Study the drawing (mm; zero at the part's minimum x, y, z) and answer. A direction names the side the tool comes from. Coordinates: 2 decimals unless noted, no trailing zeros. Order: outer loops, then holes, each group sorted by start corner. A loop starts at its lowest first (then second) coordinate and runs counter-clockwise, first axis right, second up. Notation, with made-up numbers: (25.5, 6) - (80.5, 6) arc R25 ccw to (80.5, 19) - close; hole circle Ø11 at (45, 46). An arc over 180 degrees is marked (long way). Write item = value, one per line.
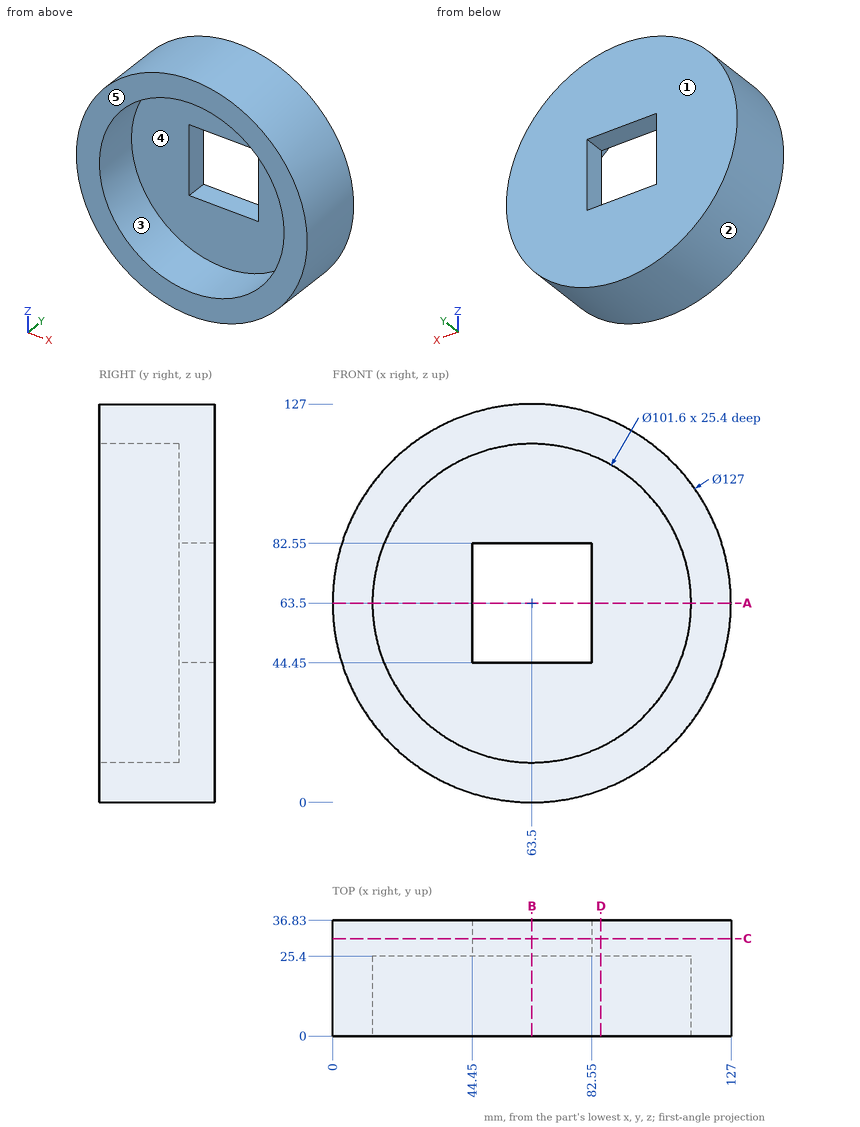
1) The part is cut by section A-A (z = 63.5). Determine the outline of the cut face in (x, y).
Returned:
outline = (0, 0) - (12.7, 0) - (12.7, 25.4) - (44.45, 25.4) - (44.45, 36.83) - (0, 36.83) - close; (82.55, 25.4) - (114.3, 25.4) - (114.3, 0) - (127, 0) - (127, 36.83) - (82.55, 36.83) - close
2) Straight lines are drawn through the part: line 1 along Z through (x, y) = (63.5, 11); line 2 along X through (y, z) = (12, 99). For each, find the intervals that lie inside material, in ascending order. Write a range as from..to.
Returned:
line_1 = 0..12.7, 114.3..127
line_2 = 10.85..27.16, 99.84..116.15
3) Flat-ended cylindrical pins translate along their axes: pin 1 Ø10 at (y, z) = (10, 51.5) entering from -X; pin 2 Ø3.5 at (y, z) = (28.5, 69.5) entering from -X; pin 3 Ø5.5 at (x, y) = (58.5, 33.5) entering from +Z. Find the tip coordinate at first contact, or state that the pin passes through.
Returned:
pin_1 = 0.39
pin_2 = 0.14
pin_3 = 126.96
4) For the marked faces 4 and 5, determine the directions among +Z, -Z, +X, -X, +Y, -Y from which every point of the face is accessible in a straight line to the end or side of a thin tool.
Returned:
face_4 = -Y
face_5 = +Z, -Z, +X, -X, -Y
5) Determine the mould class of the marked faces 1, 2 and 3 for opening direction X: pulls with the +X half, pulls with the -X half, needs draft (parallel to the pull), parting line crosses it, or undercut.
Returned:
face_1 = needs draft
face_2 = parting line crosses it
face_3 = undercut
6) The part is cut by section C-C (y = 31). Determine the outline of the cut face in (x, z), and give its area (3 significant figures).
Returned:
outline = circle Ø127 at (63.5, 63.5); hole (44.45, 44.45) - (82.55, 44.45) - (82.55, 82.55) - (44.45, 82.55) - close
area = 11,200 mm^2
7) The part is cut by section D-D (x = 85.5). Determine the outline of the cut face in (y, z).
Returned:
outline = (0, 3.93) - (36.83, 3.93) - (36.83, 123.07) - (0, 123.07) - (0, 109.29) - (25.4, 109.29) - (25.4, 17.71) - (0, 17.71) - close
8) The part is cut by section B-B (x = 63.5). Determine the outline of the cut face in (y, z), and give its area (3 significant figures).
Returned:
outline = (0, 0) - (36.83, 0) - (36.83, 44.45) - (25.4, 44.45) - (25.4, 12.7) - (0, 12.7) - close; (0, 114.3) - (25.4, 114.3) - (25.4, 82.55) - (36.83, 82.55) - (36.83, 127) - (0, 127) - close
area = 1,660 mm^2
